from build123d import *

# Parameters (mm, degrees)
SKETCH1_W                      = 152.4
SKETCH1_H                      = 76.2
BOSS_EXTRUDE1_DEPTH            = 19.05
CONVERT_SOLID1_START           = -74.5236
CONVERT_SOLID1_DEPTH           = 72.8472
CONVERT_SOLID1_START_2         = -77
CONVERT_SOLID1_2_DEPTH         = 2.273736392
CONVERT_SOLID1_START_3         = -1.473736392
CONVERT_SOLID1_3_DEPTH         = 2.473736392
CONVERT_SOLID1_START_4         = -74.726263608
CONVERT_SOLID1_4_DEPTH         = 73.252527216
CONVERT_SOLID1_5_DEPTH         = 0.202663608
CONVERT_SOLID1_START_5         = -1.6764
CONVERT_SOLID1_6_DEPTH         = 0.202663608
CONVERT_SOLID1_START_6         = 1.473736392
CONVERT_SOLID1_7_DEPTH         = 149.452527216
EDGE_FLANGE1_STRIP_W           = 5.1308
EDGE_FLANGE1_STRIP_H           = 0.889
EDGE_FLANGE1_STRIP_CUT_DEPTH   = 149.452527217
EDGE_FLANGE1_STRIP_2_W         = 5.1308
EDGE_FLANGE1_STRIP_2_H         = 0.889
EDGE_FLANGE1_STRIP_CUT_2_DEPTH = 149.452527217
EDGE_FLANGE1_DEPTH             = 149.452527217
EDGE_FLANGE1_BEND_DEPTH        = 149.452527217


with BuildPart() as part:
    # Sketch1 → Boss-Extrude1 (new body)
    with BuildSketch(Plane(origin=(0, 0, 0), x_dir=(1, 0, 0), z_dir=(0, 1, 0))):
        with Locations((76.2, 38.1)):
            Rectangle(SKETCH1_W, SKETCH1_H)
    extrude(amount=BOSS_EXTRUDE1_DEPTH)

    # Convert-Solid1: read off the stored shape, not the designer's step
    # Convert-Solid1 outline → Convert-Solid1 (cut)
    with BuildSketch(Plane.XY.offset(CONVERT_SOLID1_START)):
        with BuildLine():
            Line((151.511, 19.05), (0.889, 19.05))
            Line((0.889, 19.05), (0.889, 1.6764))
            ThreePointArc((0.889, 1.6764), (1.11962412, 1.11962412), (1.6764, 0.889))
            Line((1.6764, 0.889), (150.7236, 0.889))
            ThreePointArc((150.7236, 0.889), (151.28037588, 1.11962412), (151.511, 1.6764))
            Line((151.511, 1.6764), (151.511, 19.05))
        make_face()
        with BuildLine():
            ThreePointArc((152.4, 1.6764), (151.908993808, 0.491006192), (150.7236, 0))
            Line((150.7236, 0), (152.4, 0))
            Line((152.4, 0), (152.4, 1.6764))
        make_face()
        with BuildLine():
            Line((0, 0), (1.6764, 0))
            ThreePointArc((1.6764, 0), (0.491006192, 0.491006192), (0, 1.6764))
            Line((0, 1.6764), (0, 0))
        make_face()
    extrude(amount=CONVERT_SOLID1_DEPTH, mode=Mode.SUBTRACT)

    # Convert-Solid1 2 outline → Convert-Solid1 2 (cut)
    with BuildSketch(Plane.XY.offset(CONVERT_SOLID1_START_2)):
        Polygon((150.926263608, 2.11106664), (150.7236, 2.11106664), (150.7236, 0), (152.4, 0), (152.4, 19.05), (150.926263608, 19.05), align=None)
        Polygon((1.473736392, 19.05), (0, 19.05), (0, 0), (1.6764, 0), (1.6764, 2.11106664), (1.473736392, 2.11106664), align=None)
    extrude(amount=CONVERT_SOLID1_2_DEPTH, mode=Mode.SUBTRACT)

    # Convert-Solid1 3 outline → Convert-Solid1 3 (cut)
    with BuildSketch(Plane.XY.offset(CONVERT_SOLID1_START_3)):
        Polygon((150.926263608, 2.11106664), (150.7236, 2.11106664), (150.7236, 0), (152.4, 0), (152.4, 19.05), (150.926263608, 19.05), align=None)
        Polygon((1.473736392, 19.05), (0, 19.05), (0, 0), (1.6764, 0), (1.6764, 2.11106664), (1.473736392, 2.11106664), align=None)
    extrude(amount=CONVERT_SOLID1_3_DEPTH, mode=Mode.SUBTRACT)

    # Convert-Solid1 4 outline → Convert-Solid1 4 (cut)
    with BuildSketch(Plane.XY.offset(CONVERT_SOLID1_START_4)):
        with BuildLine():
            Line((150.926263608, 2.11106664), (150.7236, 2.11106664))
            Line((150.7236, 2.11106664), (150.7236, 0.889))
            ThreePointArc((150.7236, 0.889), (151.28037588, 1.11962412), (151.511, 1.6764))
            Line((151.511, 1.6764), (151.511, 19.05))
            Line((151.511, 19.05), (150.926263608, 19.05))
            Line((150.926263608, 19.05), (150.926263608, 2.11106664))
        make_face()
        with BuildLine():
            ThreePointArc((152.4, 1.6764), (151.908993808, 0.491006192), (150.7236, 0))
            Line((150.7236, 0), (152.4, 0))
            Line((152.4, 0), (152.4, 1.6764))
        make_face()
        with BuildLine():
            ThreePointArc((0.889, 1.6764), (1.11962412, 1.11962412), (1.6764, 0.889))
            Line((1.6764, 0.889), (1.6764, 2.11106664))
            Line((1.6764, 2.11106664), (1.473736392, 2.11106664))
            Line((1.473736392, 2.11106664), (1.473736392, 19.05))
            Line((1.473736392, 19.05), (0.889, 19.05))
            Line((0.889, 19.05), (0.889, 1.6764))
        make_face()
        with BuildLine():
            Line((0, 0), (1.6764, 0))
            ThreePointArc((1.6764, 0), (0.491006192, 0.491006192), (0, 1.6764))
            Line((0, 1.6764), (0, 0))
        make_face()
    extrude(amount=CONVERT_SOLID1_4_DEPTH, mode=Mode.SUBTRACT)

    # Convert-Solid1 5 outline → Convert-Solid1 5 (cut)
    with BuildSketch(Plane.XY.offset(CONVERT_SOLID1_START_4)):
        with BuildLine():
            ThreePointArc((151.511, 1.6764), (151.28037588, 1.11962412), (150.7236, 0.889))
            Line((150.7236, 0.889), (150.7236, 0))
            ThreePointArc((150.7236, 0), (151.908993808, 0.491006192), (152.4, 1.6764))
            Line((152.4, 1.6764), (152.4, 2.11106664))
            Line((152.4, 2.11106664), (151.511, 2.11106664))
            Line((151.511, 2.11106664), (151.511, 1.6764))
        make_face()
        with BuildLine():
            Line((1.6764, 0), (1.6764, 0.889))
            ThreePointArc((1.6764, 0.889), (1.11962412, 1.11962412), (0.889, 1.6764))
            Line((0.889, 1.6764), (0.889, 2.11106664))
            Line((0.889, 2.11106664), (0, 2.11106664))
            Line((0, 2.11106664), (0, 1.6764))
            ThreePointArc((0, 1.6764), (0.491006192, 0.491006192), (1.6764, 0))
        make_face()
    extrude(amount=CONVERT_SOLID1_5_DEPTH, mode=Mode.SUBTRACT)

    # Convert-Solid1 6 outline → Convert-Solid1 6 (cut)
    with BuildSketch(Plane.XY.offset(CONVERT_SOLID1_START_5)):
        with BuildLine():
            ThreePointArc((151.511, 1.6764), (151.28037588, 1.11962412), (150.7236, 0.889))
            Line((150.7236, 0.889), (150.7236, 0))
            ThreePointArc((150.7236, 0), (151.908993808, 0.491006192), (152.4, 1.6764))
            Line((152.4, 1.6764), (152.4, 2.11106664))
            Line((152.4, 2.11106664), (151.511, 2.11106664))
            Line((151.511, 2.11106664), (151.511, 1.6764))
        make_face()
        with BuildLine():
            Line((1.6764, 0), (1.6764, 0.889))
            ThreePointArc((1.6764, 0.889), (1.11962412, 1.11962412), (0.889, 1.6764))
            Line((0.889, 1.6764), (0.889, 2.11106664))
            Line((0.889, 2.11106664), (0, 2.11106664))
            Line((0, 2.11106664), (0, 1.6764))
            ThreePointArc((0, 1.6764), (0.491006192, 0.491006192), (1.6764, 0))
        make_face()
    extrude(amount=CONVERT_SOLID1_6_DEPTH, mode=Mode.SUBTRACT)

    # Convert-Solid1 7 outline → Convert-Solid1 7 (cut)
    with BuildSketch(Plane.YZ.offset(CONVERT_SOLID1_START_6)):
        with BuildLine():
            Line((0, 0), (0, -1.6764))
            ThreePointArc((0, -1.6764), (0.491006192, -0.491006192), (1.6764, 0))
            Line((1.6764, 0), (0, 0))
        make_face()
        with BuildLine():
            ThreePointArc((1.6764, -76.2), (0.491006192, -75.708993808), (0, -74.5236))
            Line((0, -74.5236), (0, -76.2))
            Line((0, -76.2), (1.6764, -76.2))
        make_face()
        with BuildLine():
            Line((19.05, -74.5236), (0.889, -74.5236))
            ThreePointArc((0.889, -74.5236), (1.11962412, -75.08037588), (1.6764, -75.311))
            Line((1.6764, -75.311), (19.05, -75.311))
            Line((19.05, -75.311), (19.05, -74.5236))
        make_face()
        with BuildLine():
            Line((0.889, -1.6764), (19.05, -1.6764))
            Line((19.05, -1.6764), (19.05, -0.889))
            Line((19.05, -0.889), (1.6764, -0.889))
            ThreePointArc((1.6764, -0.889), (1.11962412, -1.11962412), (0.889, -1.6764))
        make_face()
    extrude(amount=CONVERT_SOLID1_7_DEPTH, mode=Mode.SUBTRACT)

    # Edge-Flange1: sheet metal written as solids
    # Edge-Flange1 strip (on a plane across the edge) → Edge-Flange1 strip cut (cut)
    with BuildSketch(Plane(origin=(150.926263608, 19.05, 0), x_dir=(0, -1, 0), z_dir=(-1, 0, 0))):
        with Locations((-1.778, -0.4445)):
            Rectangle(EDGE_FLANGE1_STRIP_W, EDGE_FLANGE1_STRIP_H)
    extrude(amount=EDGE_FLANGE1_STRIP_CUT_DEPTH, mode=Mode.SUBTRACT)

    # Edge-Flange1 strip 2 (on a plane across the edge) → Edge-Flange1 strip cut 2 (cut)
    with BuildSketch(Plane(origin=(1.473736392, 19.05, -76.2), x_dir=(0, -1, 0), z_dir=(1, 0, 0))):
        with Locations((-1.778, -0.4445)):
            Rectangle(EDGE_FLANGE1_STRIP_2_W, EDGE_FLANGE1_STRIP_2_H)
    extrude(amount=EDGE_FLANGE1_STRIP_CUT_2_DEPTH, mode=Mode.SUBTRACT)

    # Edge-Flange1 section (on a plane across the edge) → Edge-Flange1 (add)
    with BuildSketch(Plane(origin=(150.926263608, 19.05, 0), x_dir=(0, -1, 0), z_dir=(-1, 0, 0))):
        with BuildLine():
            Line((-0.889, 0.7874), (-0.889, 11.811))
            Line((-0.889, 11.811), (0, 11.811))
            Line((0, 11.811), (0, 0.7874))
            ThreePointArc((0, 0.7874), (0.23062412, 0.23062412), (0.7874, 0))
            Line((0.7874, 0), (0.7874, -0.889))
            ThreePointArc((0.7874, -0.889), (-0.397993808, -0.397993808), (-0.889, 0.7874))
        make_face()
    extrude(amount=EDGE_FLANGE1_DEPTH)

    # Edge-Flange1 section 2 (on a plane across the edge) → Edge-Flange1 bend (add)
    with BuildSketch(Plane(origin=(1.473736392, 19.05, -76.2), x_dir=(0, -1, 0), z_dir=(1, 0, 0))):
        with BuildLine():
            Line((-0.889, 0.7874), (-0.889, 11.811))
            Line((-0.889, 11.811), (0, 11.811))
            Line((0, 11.811), (0, 0.7874))
            ThreePointArc((0, 0.7874), (0.23062412, 0.23062412), (0.7874, 0))
            Line((0.7874, 0), (0.7874, -0.889))
            ThreePointArc((0.7874, -0.889), (-0.397993808, -0.397993808), (-0.889, 0.7874))
        make_face()
    extrude(amount=EDGE_FLANGE1_BEND_DEPTH)


solid = part.part
Work out the finished part from the listing and answer in its coordinate system (mm). A direction names the side the tool comes from. Give positions to 0.01 mm unless a question says otherwise; leave off trailing zeros. Loops run counter-clockwise (first coordinate to the right, second up) from the corner with the lowest first, then second, coordinate; pieces in that order, holes last. Notation, with made-up numbers: (72.5, 31.5) - (111.5, 31.5) arc R27 ccw to (111.5, 63.5) - close; hole circle Ø2 at (88, 49). An arc over 180 degrees is marked (long way). Answer in a Markdown table with one row per item.
(1) Consider L1, parallel to X at y = 8, z = -45; L2, parallel to Z at x = 145, y = 16.25; L3, parallel to Y at x = 41, z = -31.5. Determine where each line is inside the solid, lowest interval first. Write a range as [from, to].
Results list:
| item | result |
|---|---|
| L1 | x = [0, 0.89], [151.51, 152.4] |
| L2 | z = [-76.2, -75.31], [-0.89, 0] |
| L3 | y = [0, 0.89] |
(2) Section A-A (y = 7) is taken. Give the vertices of the cut face in (x, z), and give its area (3 significant figures).
Results list:
| item | result |
|---|---|
| outline | (0, -74.73) - (0.89, -74.73) - (0.89, -1.47) - (0, -1.47) - close; (1.47, -76.2) - (150.93, -76.2) - (150.93, -75.31) - (1.47, -75.31) - close; (1.47, -0.89) - (150.93, -0.89) - (150.93, 0) - (1.47, 0) - close; (151.51, -74.73) - (152.4, -74.73) - (152.4, -1.47) - (151.51, -1.47) - close |
| area | 396 mm² |
(3) Flat-ended cylindrical pins translate along their axes: pin 1 Ø1 at (x, y) = (21, 17.5) entering from -Z; pin 2 Ø4 at (x, z) = (88, -47) entering from +Y; pin 3 Ø10 at (y, z) = (7.5, 4.5) entering from -X. Find the tip coordinate at first contact, or state that the pin passes through.
Results list:
| item | result |
|---|---|
| pin 1 | stops at z = -76.2 |
| pin 2 | stops at y = 0.89 |
| pin 3 | stops at x = 1.47 |
(4) A tool of negligible diameter and unlimited length cuts with its end or side. For faces 1 (the face through (75, 0.889, -39)), 2 (the face through (75, 19.05, -83)), 3 (the face through (151.511, 10, -39)), 4 (the face through (77, 19.05, 6)), from which of +Z, -Z, +X, -X, +Y, -Y can it reach the whole face along a straight path? Write none if from no direction.
Results list:
| item | result |
|---|---|
| face 1 | +Y |
| face 2 | -Z, +X, -X, -Y |
| face 3 | +Z, -Z, +Y |
| face 4 | +Z, +X, -X, -Y |
(5) Section B-B (z = -42) is taken. Give the vertices of the cut face in (x, y).
Results list:
| item | result |
|---|---|
| outline | (0, 1.68) arc R1.68 ccw to (1.68, 0) - (150.72, 0) arc R1.68 ccw to (152.4, 1.68) - (152.4, 19.05) - (151.51, 19.05) - (151.51, 1.68) arc R0.79 cw to (150.72, 0.89) - (1.68, 0.89) arc R0.79 cw to (0.89, 1.68) - (0.89, 19.05) - (0, 19.05) - close |
(6) For a pull along Z with two mould halves and no side action, classify faces 5 (the face through (75, 10, -0.889)), 6 (the face through (75, 19.939, -82)), 7 (the face through (75, 10, -75.311)), 8 (the face through (75, 10, 0)) as pulls with the +Z half, pulls with the -Z half, needs draft (parallel to the pull), parting line crosses it, or undercut.
Results list:
| item | result |
|---|---|
| face 5 | undercut |
| face 6 | needs draft |
| face 7 | undercut |
| face 8 | pulls with the +Z half |
(7) Section C-C (x = 87.5) is taken. Give the vertices of the cut face in (y, z), and give its area (3 significant figures).
Results list:
| item | result |
|---|---|
| outline | (0, -74.52) arc R1.68 ccw to (1.68, -76.2) - (18.26, -76.2) arc R0.79 cw to (19.05, -76.99) - (19.05, -88.01) - (19.94, -88.01) - (19.94, -76.99) arc R1.68 ccw to (18.26, -75.31) - (1.68, -75.31) arc R0.79 cw to (0.89, -74.52) - (0.89, -1.68) arc R0.79 cw to (1.68, -0.89) - (18.26, -0.89) arc R1.68 ccw to (19.94, 0.79) - (19.94, 11.81) - (19.05, 11.81) - (19.05, 0.79) arc R0.79 cw to (18.26, 0) - (1.68, 0) arc R1.68 ccw to (0, -1.68) - close |
| area | 121 mm² |
